For this review, use the dimensioned drawing (mm, ordinates from the lowest corner) and the shaded views. A direction names the side the tool comes from. Give positions to 0.01 mm unless a question says otherwise; leave off trailing zeros. Loops run counter-clockwise (first coordinate to the right, second up) from the corner with the lowest first, then second, coordinate; pieces in that order, holes last. Notation, with made-up numbers: (52, -16.5) - (87, -16.5) arc R20 ccw to (87, -6.5) - close; hole circle Ø7 at (83.25, 15). An arc over 180 degrees is marked (long way). Write each question's results on one line, items separated by ' | '.
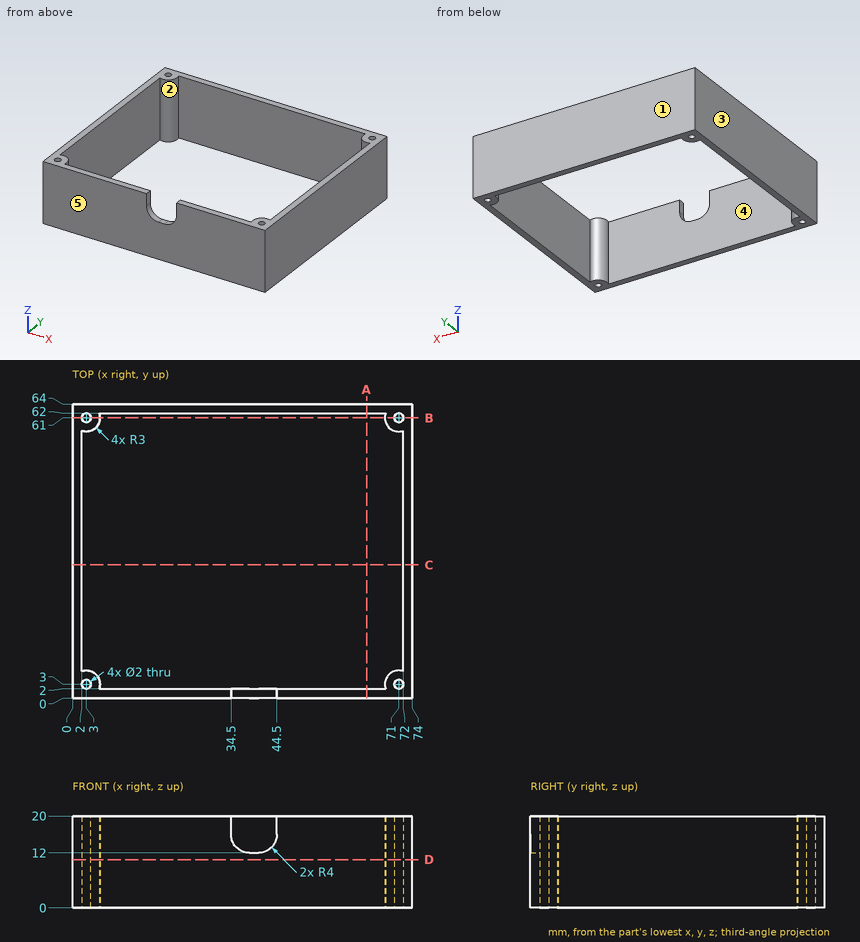
Item 1: Draft analysis for pull direction X (two halves, no side actions). For the marked faces 1, 2 and 3, state which applies: +X half, -X half, draft (parallel to the pull), parting line (faces both ways), or undercut.
Output values:
face 1: draft | face 2: undercut | face 3: -X half
Item 2: Clearance check with flat-ended pins moving along their axes: P1, Ø6, axis at x = 61, z = 4.5, coming from the -Y side; P2, Ø2, axis at x = 40, y = 1.5, coming from the +Z side. State where each tip first meets the part, or that it passes through.
Output values:
P1: stops at y = 0 | P2: stops at z = 12.03
Item 3: Wall thickness on probe 1 along Y at (x, z) = (71, 6); probe 2 along X at (y, z) = (61, 15); probe 3 along X at (y, z) = (37.5, 18.75): over which ranges is each line inside the solid? List them lowest first.
Output values:
probe 1: y = 0 to 2, 4 to 6, 58 to 60, 62 to 64 | probe 2: x = 0 to 2, 4 to 6, 68 to 70, 72 to 74 | probe 3: x = 0 to 2, 72 to 74
Item 4: We need section B-B on y = 61. Give the boundary of the cut face in (x, z).
Output values:
outline: (0, 0) - (2, 0) - (2, 20) - (0, 20) - close; (4, 0) - (6, 0) - (6, 20) - (4, 20) - close; (68, 0) - (70, 0) - (70, 20) - (68, 20) - close; (72, 0) - (74, 0) - (74, 20) - (72, 20) - close
Item 5: We need section C-C on y = 29. Give the boundary of the cut face in (x, z).
Output values:
outline: (0, 0) - (2, 0) - (2, 20) - (0, 20) - close; (72, 0) - (74, 0) - (74, 20) - (72, 20) - close
Item 6: We need section A-A on x = 64. Give the boundary of the cut face in (y, z).
Output values:
outline: (0, 0) - (2, 0) - (2, 20) - (0, 20) - close; (62, 0) - (64, 0) - (64, 20) - (62, 20) - close
Item 7: Tool access review of the marked faces 4 and 5: name each direction out of +Z, -Z, +X, -X, +Y, -Y from which nothing blocks a thin tool from reaching the whole face with its end or side.
Output values:
face 4: +Z, -Z | face 5: +Z, -Z, +X, -X, -Y
Item 8: We need section D-D on z = 10.5. Give the boundary of the cut face in (x, y).
Output values:
outline: (0, 0) - (74, 0) - (74, 64) - (0, 64) - close; hole circle Ø2 at (3, 3); hole (2, 5.83) arc R3 cw to (5.83, 2) - (68.17, 2) arc R3 cw to (72, 5.83) - (72, 58.17) arc R3 cw to (68.17, 62) - (5.83, 62) arc R3 cw to (2, 58.17) - close; hole circle Ø2 at (3, 61); hole circle Ø2 at (71, 3); hole circle Ø2 at (71, 61)
